Geometry: final body of the model. Coordinates: model frame, mm. Give positions to 0.01 mm unless a question says otherwise; leave off trailing zeros. Write each loop counter-clockwise with the first axis right and the second up, starting at its lowest first coordinate (ties: lowest second). Pieces come first, ordered by that corner, then holes.
Q1. Line query: L1, parallel to Z at x = 4.5, y = 0.75; L2, parallel to Y at x = -1, z = 31.5; L3, parallel to Y at x = 0.25, z = 22.5. Output: solid intervals per line, ascending.
Q2. Pin query (flat end, axial travel): pin 1 (4 mm diameter, centred on y = -1, z = 18, fed in from -X); pin 2 (4 mm diameter, centred on y = -2, z = 84.5, fed in from +X); pin 3 (6 mm diameter, centred on x = -1, z = 43, fed in from -Y). Return the tip coordinate at first contact, or that it passes through.
Q3. Cut plane C-C on z = 7. Return the cut outline in (x, y).
Q4. Cut plane D-D on y = -3.75. Return the cut outline in (x, z), plus the area to 3 significant figures.
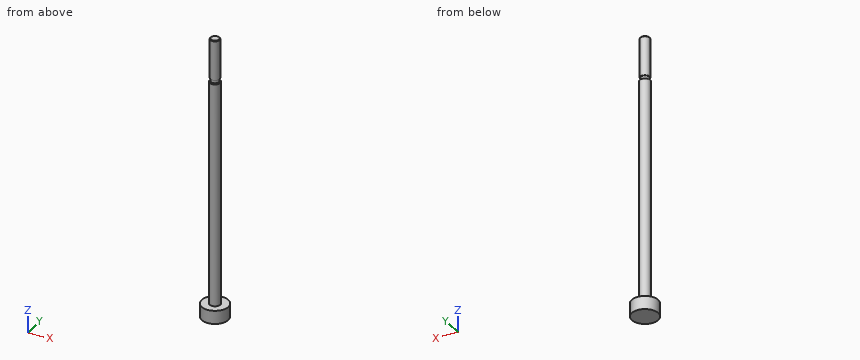
```python
from build123d import *

# Parameters (mm, degrees)
SKETCH1_R          = 2
BASE_EXTRUDE_DEPTH = 103.185
SKETCH2_R          = 5
PISTON_DEPTH       = 2.5


with BuildPart() as part:
    # Sketch1 → Base-Extrude (new body)
    with BuildSketch(Plane.XY):
        Circle(SKETCH1_R)
    extrude(amount=BASE_EXTRUDE_DEPTH)

    # Sketch2 → Piston (add, symmetric)
    with BuildSketch(Plane.XY):
        Circle(SKETCH2_R)
    extrude(amount=PISTON_DEPTH, both=True)

    # Sketch3 → Threads (revolve, cut)
    with BuildSketch(Plane(origin=(0, 0, 0), x_dir=(0, 0, -1), z_dir=(1, 0, 0))):
        Polygon((-103.185, 1.5525), (-102.985, 1.7525), (-88.185, 1.7525), (-88.185, 1.55), (-86.985, 1.55), (-86.785, 1.75), (-86.785, 5), (-103.185, 5), align=None)
    revolve(axis=Axis((0, 0, 0), (0, 0, 1)), mode=Mode.SUBTRACT)


solid = part.part
```
Data:
1. L1: z = -2.5 to 2.5
1. L2: y = -1.73 to 1.73
1. L3: y = -1.98 to 1.98
2. pin 1: stops at x = -2
2. pin 2: stops at x = 2
2. pin 3: stops at y = -2
3. outline: circle Ø4 at (0, 0)
4. outline: (-3.31, -2.5) - (3.31, -2.5) - (3.31, 2.5) - (-3.31, 2.5) - close
4. area: 33.1 mm2
